```python
from build123d import *

# Parameters (mm, degrees)
EXTRUDE_1_DEPTH     = 7.9
SKETCH_20_W         = 35
SKETCH_20_H         = 4
EXTRUDE_10_DEPTH    = 5
SKETCH_21_R         = 11
CUT_EXTRUDE_2_DEPTH = 8.9
SKETCH_2_R          = 5.341015389
CUT_EXTRUDE_3_DEPTH = 10
CUT_EXTRUDE_4_DEPTH = 3.4


with BuildPart() as part:
    # Эскиз1 → Бобышка-Вытянуть1 (new body)
    with BuildSketch(Plane(origin=(0, 0, 0), x_dir=(1, 0, 0), z_dir=(0, 1, 0))):
        with BuildLine():
            Line((191.577559736, 55.5), (0, 55.5))
            ThreePointArc((0, 55.5), (-39.244426356, -39.244426356), (55.5, 0))
            Line((55.5, 0), (191.577559736, 0))
            ThreePointArc((191.577559736, 0), (229, 27.75), (191.577559736, 55.5))
        make_face()
    extrude(amount=EXTRUDE_1_DEPTH)

    # Эскиз20 → Бобышка-Вытянуть10 (add)
    with BuildSketch(Plane(origin=(0, 7.9, 0), x_dir=(1, 0, 0), z_dir=(0, 1, 0))):
        with Locations((146.5, 51.980071838)):
            Rectangle(SKETCH_20_W, SKETCH_20_H)
    extrude(amount=EXTRUDE_10_DEPTH)

    # Эскиз21 → Вырез-Вытянуть2 (cut, through all)
    with BuildSketch(Plane(origin=(0, 7.9, 0), x_dir=(1, 0, 0), z_dir=(0, 1, 0))):
        with Locations((199.92, 27.749938535)):
            Circle(SKETCH_21_R)
    extrude(amount=-CUT_EXTRUDE_2_DEPTH, mode=Mode.SUBTRACT)

    # Эскиз2 → Вырез-Вытянуть3 (cut)
    with BuildSketch(Plane(origin=(0, 7.9, 0), x_dir=(1, 0, 0), z_dir=(0, 1, 0))):
        Circle(SKETCH_2_R)
    extrude(amount=-CUT_EXTRUDE_3_DEPTH, mode=Mode.SUBTRACT)

    # Эскиз22 → Вырез-Вытянуть4 (cut)
    with BuildSketch(Plane(origin=(0, 7.9, 0), x_dir=(1, 0, 0), z_dir=(0, 1, 0))):
        Polygon((0, 7.1), (-6.148780367, 3.55), (-6.148780367, -3.55), (0, -7.1), (6.148780367, -3.55), (6.148780367, 3.55), align=None)
    extrude(amount=-CUT_EXTRUDE_4_DEPTH, mode=Mode.SUBTRACT)


solid = part.part
```
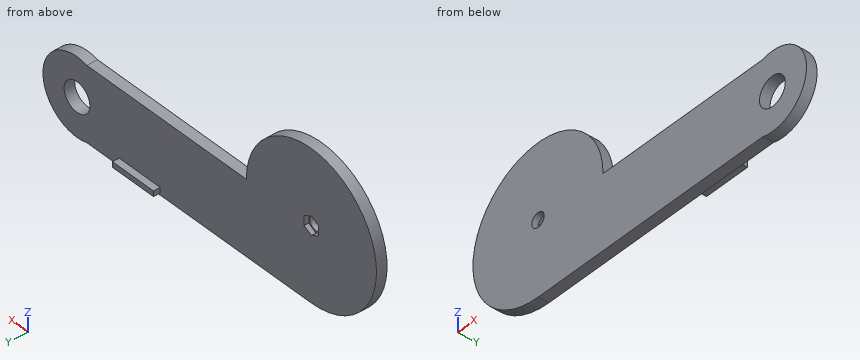
Could you check a few things on this model? Use its own coordinates, in mm. Round coordinates to 2 decimals unless told otherwise and drop trailing zeros. Loops run counter-clockwise (first coordinate to the right, second up) from the corner with the lowest first, then second, coordinate; pieces in that order, holes last.
Q1. For P1, Ø1.5, axis at y = 5.5, z = -36.5, coming from the -X side; P2, Ø5.5, axis at x = 138, y = 10.5, coming from the +Z side; P3, Ø4, axis at x = 143, y = 11.5, coming from the -Z side, each with a flat end and sliding along its axis, tell me the tip position at first contact or that it passes through.
Q2. I want a section at D-D (x = -30). Write out the boundary of the cut face in (y, z), and give its area (3 significant figures).
Q3. I want a section at A-A (x = 199.92). Write out the boundary of the cut face in (y, z), and give its area (3 significant figures).
Q4. I want a section at B-B (x = 140). Write out the boundary of the cut face in (y, z).
Q5. I want a section at C-C (z = 45). Write out the boundary of the cut face in (x, y).
Q6. Please list where these lines run through material, in increasing order: L1, parallel to Z at x = 199.92, y = 1.5; L2, parallel to Z at x = 0, y = 2.5; L3, parallel to Y at x = 53, z = -2.
Answer below:
1. P1: stops at x = -42.45
1. P2: stops at z = 0
1. P3: stops at z = -53.98
2. outline: (0, -46.69) - (7.9, -46.69) - (7.9, 46.69) - (0, 46.69) - close
2. area: 738 mm2
3. outline: (0, -56.75) - (7.9, -56.75) - (7.9, -38.75) - (0, -38.75) - close; (0, -16.75) - (7.9, -16.75) - (7.9, 1.25) - (0, 1.25) - close
3. area: 284 mm2
4. outline: (0, -55.5) - (7.9, -55.5) - (7.9, -53.98) - (12.9, -53.98) - (12.9, -49.98) - (7.9, -49.98) - (7.9, 0) - (0, 0) - close
5. outline: (-32.48, 0) - (32.48, 0) - (32.48, 7.9) - (-32.48, 7.9) - close
6. L1: z = -56.75 to -38.75, -16.75 to 1.25
6. L2: z = -55.5 to -5.34, 5.34 to 55.5
6. L3: y = 0 to 7.9
